Autodesk Inventor part; units mm, degrees
ref_plane "YZ Plane" through (0, 0, 0) normal (1, 0, 0) x (0, 1, 0)
ref_plane "XZ Plane" through (0, 0, 0) normal (0, 1, 0) x (-1, 0, 0)
ref_plane "XY Plane" through (0, 0, 0) normal (0, 0, 1) x (1, 0, 0)
sketch "Schizzo1" plane through (0, 0, 0) normal (0, 0, 1) x (1, 0, 0)
  circle A0 centre (0, 0) radius 4.5
  dimension "d0" = 9
extrude "Estrusione1" add sketch "Schizzo1" along normal mid plane 53
sketch "Schizzo2" plane through (0, 0, 26.5) normal (0, 0, 1) x (1, 0, 0)
  circle A0 centre (0, 0) radius 4.5
  circle A1 centre (0, 0) radius 7
  dimension "d3" = 14
extrude "Estrusione2" add sketch "Schizzo2" along normal blind 2 contours A0 | A1
chamfer "Smusso1" distance 0.5 angle 45 1 edges at (-4.5, 0, -26.5)
thread "Filettatura1"
fillet "Raccordo1" radius 0.5 2 edges at (-7, 0, 28.5) (-7, 0, 26.5)
properties part number "Kingpin"
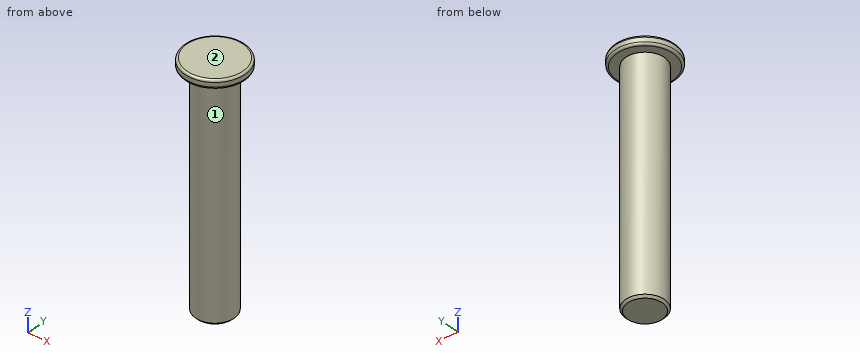
Work out the finished part from the listing and answer in its coordinate system (mm). Face numbers are marked on the shaded views. A direction names the side the tool comes from. Coordinates: 2 decimals unless noted, no trailing zeros. Loops run counter-clockwise (first coordinate to the right, second up) from the corner with the lowest first, then second, coordinate; pieces in that order, holes last. Notation, with made-up numbers: (-29.75, 33) -> (9.25, 33) arc R17 cw to (9.25, 54) -> close; hole circle Ø9 at (44.25, -37). An arc over 180 degrees is marked (long way). Write each question's results on one line, items separated by ' | '. Start each with the question number.
1) Find section A-A on x = 0. Determine the outline of the cut face in (y, z).
2) Find section C-C on z = 19. Determine the outline of the cut face in (x, y), then the cut area to 3 significant figures.
3) Flat-ended cylindrical pins translate along their axes: P1, Ø1, axis at y = 5.5, z = 12, coming from the +X side; P2, Ø3, axis at y = 4.5, z = -2.5, coming from the -X side; P3, Ø3, axis at x = 3.5, z = 5.5, coming from the +Y side. Find the tip coordinate at first contact, or state that the pin passes through.
4) For the marked faces 1 and 2, determine the directions among +Z, -Z, +X, -X, +Y, -Y from which every point of the face is accessible in a straight line to the end or side of a thin tool.
5) Consider line 1 along Z through (x, y) = (-5, 3); line 2 along Y through (x, z) = (0, -6.5); line 3 along X through (y, z) = (2.5, 17.5). Determine where each line is inside the solid, lowest interval first.
Response values:
1) outline: (-7, 27) arc R0.5 ccw to (-6.5, 26.5) -> (-4.5, 26.5) -> (-4.5, -26) -> (-4, -26.5) -> (4, -26.5) -> (4.5, -26) -> (4.5, 26.5) -> (6.5, 26.5) arc R0.5 ccw to (7, 27) -> (7, 28) arc R0.5 ccw to (6.5, 28.5) -> (-6.5, 28.5) arc R0.5 ccw to (-7, 28) -> close
2) outline: circle Ø9 at (0, 0) | area: 63.6 mm^2
3) P1: passes through | P2: stops at x = -3.35 | P3: stops at y = 4.03
4) face 1: -Z | face 2: +Z, +X, -X, +Y, -Y
5) line 1: z = 26.5 to 28.5 | line 2: y = -4.5 to 4.5 | line 3: x = -3.74 to 3.74
